Verification items for this drawing (mm, ordinates from the low corner). A direction names the side the tool comes from. Round coordinates to 2 decimals unless told otherwise and drop trailing zeros. Order: outer loops, then holes, each group sorted by start corner. A loop starts at its lowest first (then second) coordinate and runs counter-clockwise, first axis right, second up. Notation, with made-up numbers: M 62.25,1.25 L 114.25,1.25 A19 cw 114.25,19.25 Z; hole C 37.5,76.25 d10. An arc over 180 degrees is marked long. Return JSON: item names as keys, results as strings. Group by question number.
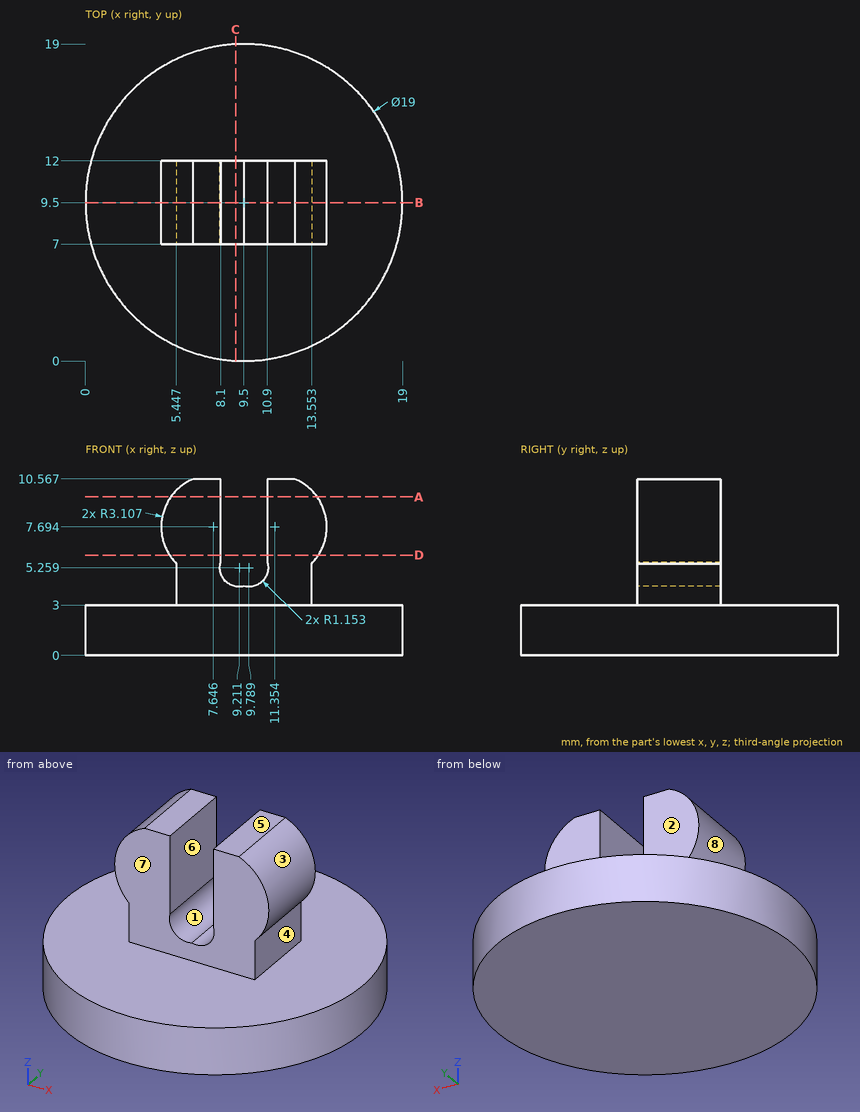
Q1. Material ranges on line 1 along Z through (x, y) = (10.75, 1.75); line 2 along Y through (x, z) = (12, 9.5); line 3 along Z through (x, y) = (13.75, 9) (1 decimal), recorded low to high.
Q2. Section check A-A on z = 9.5. Record the cut outline in (x, y), plus the area to 3 significant figures.
Q3. Release check for a two-part mould opening along X. For the marked faces 1, 2 and 3 record: +X half, -X half, draft (parallel to the pull), parting line (faces both ways), or undercut.
Q4. Section check D-D on z = 6. Record the cut outline in (x, y).
Q5. Section check C-C on x = 9. Record the cut outline in (y, z) (1 decimal).
Q6. Depth check by flat-ended pin: pin 1 Ø4 at (x, z) = (7.5, 7) entering from -Y; pin 2 Ø1.5 at (y, z) = (10, 8) entering from +X; pin 3 Ø1.5 at (y, z) = (9, 8.5) entering from -X. Enter the tip coordinate at first touch or a pass-through.
Q7. Section check B-B on y = 9.5. Record the cut outline in (x, z).
Q8. Set-up check for the marked faces 4, 5, 6, 7 and 8: record each of +Z, -Z, +X, -X, +Y, -Y from which the full face is reachable in a straight line by a thin tool's end or side.
Geometry check:
{
 "1": {"line 1": "z = 0 to 3", "line 2": "y = 7 to 12", "line 3": "z = 0 to 3, 5.7 to 9.7"},
 "2": {"outline": "M 5.12,7 L 8.1,7 L 8.1,12 L 5.12,12 Z; M 10.9,7 L 13.88,7 L 13.88,12 L 10.9,12 Z", "area": "29.8 mm^2"},
 "3": {"face 1": "undercut", "face 2": "draft", "face 3": "+X half"},
 "4": {"outline": "M 5.04,7 L 8.1,7 L 8.1,12 L 5.04,12 Z; M 10.9,7 L 13.96,7 L 13.96,12 L 10.9,12 Z"},
 "5": {"outline": "M 0,0 L 19,0 L 19,3 L 12,3 L 12,4.1 L 7,4.1 L 7,3 L 0,3 Z"},
 "6": {"pin 1": "stops at y = 7", "pin 2": "stops at x = 14.46", "pin 3": "stops at x = 4.54"},
 "7": {"outline": "M 0,0 L 19,0 L 19,3 L 13.55,3 L 13.55,5.5 A3.11 ccw 12.54,10.57 L 10.9,10.57 L 10.9,5.57 A1.15 cw 9.5,4.14 A1.15 cw 8.1,5.57 L 8.1,10.57 L 6.46,10.57 A3.11 ccw 5.45,5.5 L 5.45,3 L 0,3 Z"},
 "8": {"face 4": "+X, +Y, -Y", "face 5": "+Z, +X, -X, +Y, -Y", "face 6": "+Z, +Y, -Y", "face 7": "+Z, +X, -X, -Y", "face 8": "-X, +Y, -Y"}
}
